Read the model definition and answer for the solid it produces. Units are mm, in the model's axes. A direction names the side the tool comes from. Give positions to 0.01 mm unless a question says otherwise; leave off trailing zeros. Loops run counter-clockwise (first coordinate to the right, second up) from the corner with the lowest first, then second, coordinate; pieces in that order, holes last. Notation, with made-up numbers: (43, 79.5) - (100, 79.5) arc R9 ccw to (100, 86.5) - close; hole circle Ø6 at (-29, 59). An arc over 180 degrees is marked (long way). Put each result on its own line as item: value. Start each with the question number.
1. A cutting plane is placed at C-C, the plane z = 475. Determine the outline of the cut face in (x, y).
2. Consider L1, parallel to Y at x = 601.5, z = 536; L2, parallel to X at y = 646, z = 876; L3, parallel to Z at x = 840, y = 632.5. Determine where each line is inside the solid, lowest interval first. Write a range as from..to.
3. A cutting plane is placed at A-A, the plane y = 721. Determine the outline of the cut face in (x, z).
4. A cutting plane is placed at B-B, the plane x = 1323. Determine the outline of the cut face in (y, z), plus the area to 3 significant figures.
5. A cutting plane is placed at D-D, the plane z = 908. Determine the outline of the cut face in (x, y), plus the area to 3 significant figures.
6. For a pull along X with two mould halves and no side action, classify faces 1 (the flat face through (582, 1016, 388)), 2 (the flat face through (0, 501, 501)), 3 (the flat face through (504.441, 125.222, 765.556)), 4 (the cylindrical face through (1100.93, 332.91, 257.56)) as released by +X, released by -X, zero draft, split by the parting line, or undercut.
7. For faces 5 (the flat face through (206, 628, 1016)), 6 (the flat face through (512, 762, 766)), 7 (the flat face through (762, 891, 766)), determine the directions among +Z, -Z, +X, -X, +Y, -Y from which every point of the face is accessible in a straight line to the end or side of a thin tool.
8. Given pin 1 Ø6 at (x, y) = (868, 365.5) entering from +Z, flat-ended and moving along its own axis, determine where the tip first touches the part or whether it passes through.
```python
from build123d import *

# Parameters (mm, degrees)
F0_W     = 1778
F0_H     = 1016
F1_DEPTH = 1016
F3_DEPTH = 508
F6_DEPTH = 254
F4_W     = 508
F4_H     = 254
F7_DEPTH = 175.26
F8_R     = 254
F9_DEPTH = 508
F10_R    = 254
F11_R    = 254


with BuildPart() as f1:
    # F0 (on Top) → F1 (new body)
    with BuildSketch(Plane.XY):
        with Locations((889, 508)):
            Rectangle(F0_W, F0_H)
    extrude(amount=F1_DEPTH)

    # F2 (on face) → F3 (cut)
    with BuildSketch(Plane.XY.offset(1016)):
        Polygon((1778, 1016), (762, 1016), (762, 762), (254, 762), (254, 254), (762, 254), (762, 0), (1778, 0), align=None)
    extrude(amount=-F3_DEPTH, mode=Mode.SUBTRACT)

    # F5 (on face) → F6 (cut)
    with BuildSketch(Plane.XZ):
        Polygon((762, 1016), (253.9933919907, 1016), (762, 508), align=None)
    extrude(amount=-F6_DEPTH, mode=Mode.SUBTRACT)

    # F4 (on face) → F7 (cut)
    with BuildSketch(Plane.XY.offset(1016)):
        with Locations((508, 127)):
            Rectangle(F4_W, F4_H)
    extrude(amount=F7_DEPTH, mode=Mode.SUBTRACT)

    # F8 (on face) → F9 (cut)
    with BuildSketch(Plane.XY.offset(508)):
        with Locations((1302.4921417236, 487.4676764011)):
            Circle(F8_R)
    extrude(amount=-F9_DEPTH, mode=Mode.SUBTRACT)

    # F10
    f10_edges = [f1.edges().sort_by_distance(p)[0] for p in [
        (1778, 0, 254),
    ]]
    fillet(f10_edges, radius=F10_R)

    # F11
    f11_edges = [f1.edges().sort_by_distance(p)[0] for p in [
        (1778, 1016, 254),
    ]]
    fillet(f11_edges, radius=F11_R)


solid = f1.part
```
Return value:
1. outline: (0, 0) - (1524, 0) arc R254 ccw to (1778, 254) - (1778, 762) arc R254 ccw to (1524, 1016) - (0, 1016) - close; hole circle Ø508 at (1302.49, 487.47)
2. L1: y = 0..254, 762..1016
2. L2: x = 0..254
2. L3: z = 0..508
3. outline: (0, 0) - (1202.6, 0) - (1202.6, 508) - (254, 508) - (254, 1016) - (0, 1016) - close; (1402.39, 0) - (1778, 0) - (1778, 508) - (1402.39, 508) - close
4. outline: (0, 0) - (234.3, 0) - (234.3, 508) - (0, 508) - close; (740.64, 0) - (1016, 0) - (1016, 508) - (740.64, 508) - close
4. area: 259,000 mm2
5. outline: (0, 0) - (361.99, 0) - (361.99, 254) - (254, 254) - (254, 762) - (762, 762) - (762, 1016) - (0, 1016) - close
5. area: 415,000 mm2
6. face 1: zero draft
6. face 2: released by -X
6. face 3: released by +X
6. face 4: undercut
7. face 5: +Z, +X, -X, +Y, -Y
7. face 6: +Z, +X
7. face 7: +Z, +X, +Y, -Y
8. pin 1: stops at z = 508
